Design review of the part built by this model. Coordinates are the model's own, in mm. A direction names the side the tool comes from. Coordinates: 2 decimals unless noted, no trailing zeros. Order: outer loops, then holes, each group sorted by start corner. A loop starts at its lowest first (then second) coordinate and runs counter-clockwise, first axis right, second up. Notation, with made-up numbers: (54, -32.5) - (63, -32.5) arc R21 ccw to (63, -2.5) - close; hole circle Ø11 at (-32, 2). An arc over 180 degrees is marked (long way). Write each question's results on one line, items separated by ' | '. Start each with the question number.
```python
from build123d import *

# Parameters (mm, degrees)
BOSS_EXTRUDE8_DEPTH  = 3
CUT_EXTRUDE8_DEPTH   = 3
BOSS_EXTRUDE9_DEPTH  = 25
SKETCH17_R           = 7.5
BOSS_EXTRUDE10_DEPTH = 2
SKETCH18_R           = 1.5
CUT_EXTRUDE9_DEPTH   = 62
SKETCH19_R           = 7.5
BOSS_EXTRUDE11_DEPTH = 2
SKETCH21_R           = 1.5
CUT_EXTRUDE10_DEPTH  = 52
CUT_EXTRUDE11_DEPTH  = 22


with BuildPart() as part:
    # Sketch1 → Boss-Extrude8 (new body)
    with BuildSketch(Plane(origin=(0, 0, 0), x_dir=(1, 0, 0), z_dir=(0, 1, 0))):
        with BuildLine():
            Line((2, 0), (48, 0))
            ThreePointArc((48, 0), (49.414213562, 0.585786438), (50, 2))
            Line((50, 2), (50, 8))
            ThreePointArc((50, 8), (49.414213562, 9.414213562), (48, 10))
            Line((48, 10), (2, 10))
            ThreePointArc((2, 10), (0.585786438, 9.414213562), (0, 8))
            Line((0, 8), (0, 2))
            ThreePointArc((0, 2), (0.585786438, 0.585786438), (2, 0))
        make_face()
    extrude(amount=BOSS_EXTRUDE8_DEPTH)

    # Sketch15 → Cut-Extrude8 (cut)
    with BuildSketch(Plane(origin=(0, 3, 0), x_dir=(1, 0, 0), z_dir=(0, 1, 0))):
        with BuildLine():
            Line((3.75, 5), (5, 5))
            Line((5, 5), (6.25, 5))
            ThreePointArc((6.25, 5), (5, 6.25), (3.75, 5))
        make_face()
        with BuildLine():
            Line((6.25, 5), (5, 5))
            Line((5, 5), (3.75, 5))
            ThreePointArc((3.75, 5), (5, 3.75), (6.25, 5))
        make_face()
        with BuildLine():
            ThreePointArc((46.25, 5), (45, 6.25), (43.75, 5))
            Line((43.75, 5), (45, 5))
            Line((45, 5), (46.25, 5))
        make_face()
        with BuildLine():
            Line((45, 5), (43.75, 5))
            ThreePointArc((43.75, 5), (45, 3.75), (46.25, 5))
            Line((46.25, 5), (45, 5))
        make_face()
    extrude(amount=-CUT_EXTRUDE8_DEPTH, mode=Mode.SUBTRACT)

    # Sketch16 → Boss-Extrude9 (add)
    with BuildSketch(Plane(origin=(0, 3, 0), x_dir=(1, 0, 0), z_dir=(0, 1, 0))):
        with BuildLine():
            Line((9.25, 5), (12.25, 5))
            Line((12.25, 5), (15.25, 5))
            ThreePointArc((15.25, 5), (12.25, 8), (9.25, 5))
        make_face()
        with BuildLine():
            Line((15.25, 5), (12.25, 5))
            Line((12.25, 5), (9.25, 5))
            ThreePointArc((9.25, 5), (12.25, 2), (15.25, 5))
        make_face()
        with BuildLine():
            ThreePointArc((40.75, 5), (37.75, 8), (34.75, 5))
            Line((34.75, 5), (37.75, 5))
            Line((37.75, 5), (40.75, 5))
        make_face()
        with BuildLine():
            Line((37.75, 5), (34.75, 5))
            ThreePointArc((34.75, 5), (37.75, 2), (40.75, 5))
            Line((40.75, 5), (37.75, 5))
        make_face()
    extrude(amount=BOSS_EXTRUDE9_DEPTH)

    # Sketch17 → Boss-Extrude10 (add)
    with BuildSketch(Plane(origin=(0, 28, 0), x_dir=(1, 0, 0), z_dir=(0, 1, 0))):
        with Locations((12.25, 5)):
            Circle(SKETCH17_R)
    extrude(amount=BOSS_EXTRUDE10_DEPTH)

    # Sketch18 → Cut-Extrude9 (cut)
    with BuildSketch(Plane(origin=(0, 30, 0), x_dir=(1, 0, 0), z_dir=(0, 1, 0))):
        with Locations((12.25, 5)):
            Circle(SKETCH18_R)
    extrude(amount=-CUT_EXTRUDE9_DEPTH, mode=Mode.SUBTRACT)

    # Sketch19 → Boss-Extrude11 (add)
    with BuildSketch(Plane(origin=(0, 28, 0), x_dir=(1, 0, 0), z_dir=(0, 1, 0))):
        with Locations((37.75, 5)):
            Circle(SKETCH19_R)
    extrude(amount=BOSS_EXTRUDE11_DEPTH)

    # Sketch21 → Cut-Extrude10 (cut)
    with BuildSketch(Plane(origin=(0, 30, 0), x_dir=(1, 0, 0), z_dir=(0, 1, 0))):
        with Locations((37.75, 5)):
            Circle(SKETCH21_R)
    extrude(amount=-CUT_EXTRUDE10_DEPTH, mode=Mode.SUBTRACT)

    # Sketch23 → Cut-Extrude11 (cut)
    with BuildSketch(Plane.XZ):
        with BuildLine():
            ThreePointArc((27, -5), (25, -3), (23, -5))
            Line((23, -5), (27, -5))
        make_face()
        with BuildLine():
            Line((27, -5), (23, -5))
            ThreePointArc((23, -5), (25, -7), (27, -5))
        make_face()
    extrude(amount=-CUT_EXTRUDE11_DEPTH, mode=Mode.SUBTRACT)


solid = part.part
```
(1) Take a section at A-A (x = 37.75). State the section outline as (y, z) points, plus the area to 3 significant figures.
(2) Take a section at D-D (z = -8.75). State the section outline as (x, y) points, plus the area to 3 significant figures.
(3) To check wall thickness, follow line 1 along Z through (x, y) = (37.75, 21.5); line 2 along Z through (x, y) = (45, 1.9); line 3 along X through (y, z) = (12, -6.75). State the ranges of each line that lie inside material, in increasing order. Write a range as [from, to].
(4) Mouldability with a two-part tool opening along Y and no side actions: class faces 1 (the face through (15.5, 28, -5.1)), 2 (the face through (14.46, 15.32, -2.97)), 3 (the face through (49.43, 1.48, -9.4)), 4 (the face through (38, 30, -3)) as +Y half, -Y half, draft (parallel to the pull), parting line (faces both ways), or undercut.
(5) Take a section at C-C (z = 1.25). State the section outline as (x, y) points.
(6) Take a section at B-B (y = 18). State the section outline as (x, z) points.
(7) Clearance check with flat-ended pins moving along their axes: pin 1 (1.5 mm diameter, centred on x = 20.5, z = -1.5, fed in from -Y); pin 2 (2.5 mm diameter, centred on x = 28.5, y = 1.5, fed in from +Z); pin 3 (1 mm diameter, centred on x = 28, z = -4, fed in from +Y); pin 4 (1.5 mm diameter, centred on x = 5, z = -5, fed in from -Y). State where each tip first meets the part, or that it passes through.
(8) Tool access review of faces 5 (the face through (25, 1, -10)), 6 (the face through (37.6, 28, -1.8)), 7 (the face through (25, 1, 0)), 8 (the face through (45.99, 1.52, -5.76)), 9 (the face through (11.274, 28.986, -12.436)): name each direction out of +Z, -Z, +X, -X, +Y, -Y from which nothing blocks a thin tool from reaching the whole face with its end or side.
Worked out:
1) outline: (0, -10) - (3, -10) - (3, -8) - (28, -8) - (28, -12.5) - (30, -12.5) - (30, -6.5) - (0, -6.5) - close; (0, -3.5) - (30, -3.5) - (30, 2.5) - (28, 2.5) - (28, -2) - (3, -2) - (3, 0) - (0, 0) - close | area: 120 mm^2
2) outline: (0.15, 0) - (49.85, 0) - (49.85, 3) - (0.15, 3) - close; (5.75, 28) - (18.75, 28) - (18.75, 30) - (5.75, 30) - close; (31.25, 28) - (44.25, 28) - (44.25, 30) - (31.25, 30) - close | area: 201 mm^2
3) line 1: [-8, -6.5], [-3.5, -2] | line 2: [-10, -6.25], [-3.75, 0] | line 3: [9.81, 14.69], [35.31, 40.19]
4) face 1: undercut | face 2: undercut | face 3: draft | face 4: +Y half
5) outline: (8.1, 28) - (16.4, 28) - (16.4, 30) - (8.1, 30) - close; (33.6, 28) - (41.9, 28) - (41.9, 30) - (33.6, 30) - close
6) outline: circle Ø6 at (12.25, -5); circle Ø6 at (37.75, -5); hole circle Ø3 at (12.25, -5); hole circle Ø3 at (37.75, -5)
7) pin 1: y = 0 | pin 2: z = 0 | pin 3: y = 3 | pin 4: y = 28
8) face 5: -Z, +X, -X, -Y | face 6: none | face 7: +Z, +X, -X, -Y | face 8: -Y | face 9: +Y
